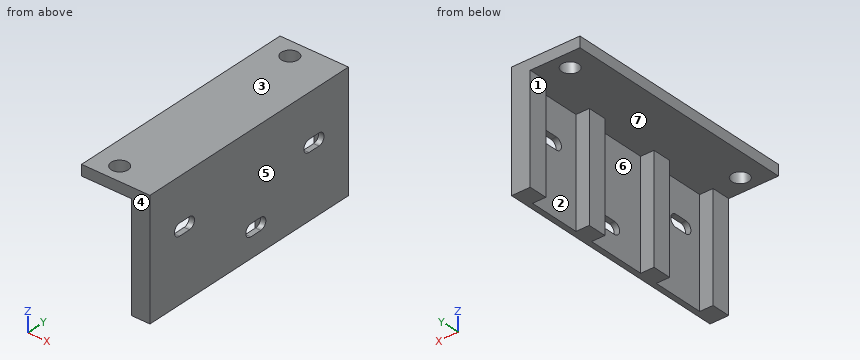
from build123d import *

# Parameters (mm, degrees)
SKETCH1_W           = 25.6624
SKETCH1_H           = 88.9
SKETCH1_R           = 3.175
BOSS_EXTRUDE1_DEPTH = 2
SKETCH2_W           = 2
SKETCH2_H           = 88.9
BOSS_EXTRUDE2_DEPTH = 40
CUT_EXTRUDE1_DEPTH  = 20
SKETCH8_W           = 40
SKETCH8_H           = 7
BOSS_EXTRUDE6_DEPTH = 5
BOSS_EXTRUDE8_START = 2
SKETCH9_W           = 25.6624
SKETCH9_H           = 88.9
SKETCH9_R           = 3.175
BOSS_EXTRUDE8_DEPTH = 2
BOSS_EXTRUDE5_START = 1
SKETCH7_W           = 25.6624
SKETCH7_H           = 88.9
SKETCH7_R           = 3.175
BOSS_EXTRUDE5_DEPTH = 1


with BuildPart() as part:
    # Sketch1 → Boss-Extrude1 (new body)
    with BuildSketch(Plane.XY):
        with Locations((3.8312, 0)):
            Rectangle(SKETCH1_W, SKETCH1_H)
        with Locations((0, -38.1)):
            Circle(SKETCH1_R, mode=Mode.SUBTRACT)
        with Locations((0, 38.1)):
            Circle(SKETCH1_R, mode=Mode.SUBTRACT)
    extrude(amount=-BOSS_EXTRUDE1_DEPTH)

    # Sketch2 → Boss-Extrude2 (add)
    with BuildSketch(Plane(origin=(0, 0, -2), x_dir=(-1, 0, 0), z_dir=(0, 0, -1))):
        with Locations((-15.6624, 0)):
            Rectangle(SKETCH2_W, SKETCH2_H)
    extrude(amount=BOSS_EXTRUDE2_DEPTH)

    # Sketch3 → Cut-Extrude1 (cut)
    with BuildSketch(Plane(origin=(16.6624, 0, 0), x_dir=(0, 0, -1), z_dir=(1, 0, 0))):
        with BuildLine():
            Line((14, -26.75), (14, -31.25))
            ThreePointArc((14, -31.25), (16.25, -33.5), (18.5, -31.25))
            Line((18.5, -31.25), (18.5, -26.75))
            ThreePointArc((18.5, -26.75), (16.25, -24.5), (14, -26.75))
        make_face()
        with BuildLine():
            Line((18.5, 26.75), (18.5, 31.25))
            ThreePointArc((18.5, 31.25), (16.25, 33.5), (14, 31.25))
            Line((14, 31.25), (14, 26.75))
            ThreePointArc((14, 26.75), (16.25, 24.5), (18.5, 26.75))
        make_face()
        with BuildLine():
            Line((30, 5.2), (30, 0.7))
            ThreePointArc((30, 0.7), (32.25, -1.55), (34.5, 0.7))
            Line((34.5, 0.7), (34.5, 5.2))
            ThreePointArc((34.5, 5.2), (32.25, 7.45), (30, 5.2))
        make_face()
    extrude(amount=-CUT_EXTRUDE1_DEPTH, mode=Mode.SUBTRACT)

    # Sketch8 → Boss-Extrude6 (add)
    with BuildSketch(Plane.ZY.offset(-14.6624)):
        with Locations((-22, -14.5)):
            Rectangle(SKETCH8_W, SKETCH8_H)
        with Locations((-22, 14.5)):
            Rectangle(SKETCH8_W, SKETCH8_H)
        with Locations((-22, 40.95)):
            Rectangle(SKETCH8_W, SKETCH8_H)
        with Locations((-22, -40.95)):
            Rectangle(SKETCH8_W, SKETCH8_H)
    extrude(amount=BOSS_EXTRUDE6_DEPTH)

    # Sketch9 → Boss-Extrude8 (add)
    with BuildSketch(Plane.XY.offset(BOSS_EXTRUDE8_START)):
        with Locations((3.8312, 0)):
            Rectangle(SKETCH9_W, SKETCH9_H)
        with Locations((0, -38.1)):
            Circle(SKETCH9_R, mode=Mode.SUBTRACT)
        with Locations((0, 38.1)):
            Circle(SKETCH9_R, mode=Mode.SUBTRACT)
    extrude(amount=-BOSS_EXTRUDE8_DEPTH)

    # Sketch7 → Boss-Extrude5 (add)
    with BuildSketch(Plane.XY.offset(BOSS_EXTRUDE5_START)):
        with Locations((3.8312, 0)):
            Rectangle(SKETCH7_W, SKETCH7_H)
        with Locations((0, -38.1)):
            Circle(SKETCH7_R, mode=Mode.SUBTRACT)
        with Locations((0, 38.1)):
            Circle(SKETCH7_R, mode=Mode.SUBTRACT)
    extrude(amount=-BOSS_EXTRUDE5_DEPTH)


solid = part.part
Could you check a few things on this model? Use its own coordinates, in mm. Face numbers are marked on the shaded views. A direction names the side the tool comes from. Give positions to 0.01 mm unless a question says otherwise; leave off trailing zeros. Order: outer loops, then holes, each group sorted by start corner. A loop starts at its lowest first (then second) coordinate and runs counter-clockwise, first axis right, second up. Notation, with made-up numbers: (66.25, 61) - (103.25, 61) arc R25 ccw to (103.25, 94) - close; hole circle Ø9 at (29, 63.5). An arc over 180 degrees is marked (long way). One line per item, written item: value. Start each with the question number.
1. For P1, Ø2, axis at y = -16, z = -12.5, coming from the -X side; P2, Ø1.5, axis at y = 23.5, z = -20, coming from the -X side; P3, Ø10, axis at x = 0, y = 38.1, coming from the -Z side, each with a flat end and sliding along its axis, tell me the tip position at first contact or that it passes through.
2. Imagine slicing it at C-C on z = -29. List the corners of the cut face in (x, y) for me.
3. Imagine slicing it at A-A on z = -16.25. List the corners of the cut face in (x, y) for me.
4. Thinking about a two-plate mould opening in Y: for the marked faces 4, 5, 6 and 7, which applies, +Y half, -Y half, draft (parallel to the pull), parting line (faces both ways), or undercut?
5. Imagine slicing it at D-D on x = 5. List the corners of the cut face in (y, z) for me, plus the area to 3 significant figures.
6. Imagine slicing it at B-B on y = -16.5. List the corners of the cut face in (x, z) for me, plus the area to 3 significant figures.
7. If I drill on probe 1 along Y at (x, z) = (0, -0.4) (3 decimals); probe 2 along Y at (x, z) = (12, -19.5); probe 3 along Y at (x, z) = (-0.5, -1), over which ranges is the centre line in solid material (lowest first)?
8. For the marked faces 1, 2 and 3, which set-ups out of +Z, -Z, +X, -X, +Y, -Y let a thin tool reach every point of the face, with its end or its side?
Values:
1. P1: x = 9.66
1. P2: x = 14.66
1. P3: z = -2
2. outline: (9.66, -44.45) - (16.66, -44.45) - (16.66, 44.45) - (9.66, 44.45) - (9.66, 37.45) - (14.66, 37.45) - (14.66, 18) - (9.66, 18) - (9.66, 11) - (14.66, 11) - (14.66, -11) - (9.66, -11) - (9.66, -18) - (14.66, -18) - (14.66, -37.45) - (9.66, -37.45) - close
3. outline: (9.66, -44.45) - (16.66, -44.45) - (16.66, -33.5) - (14.66, -33.5) - (14.66, -37.45) - (9.66, -37.45) - close; (9.66, -18) - (14.66, -18) - (14.66, -24.5) - (16.66, -24.5) - (16.66, 24.5) - (14.66, 24.5) - (14.66, 18) - (9.66, 18) - (9.66, 11) - (14.66, 11) - (14.66, -11) - (9.66, -11) - close; (9.66, 37.45) - (14.66, 37.45) - (14.66, 33.5) - (16.66, 33.5) - (16.66, 44.45) - (9.66, 44.45) - close
4. face 4: -Y half
4. face 5: draft
4. face 6: undercut
4. face 7: undercut
5. outline: (-44.45, -2) - (44.45, -2) - (44.45, 2) - (-44.45, 2) - close
5. area: 356 mm²
6. outline: (-9, -2) - (9.66, -2) - (9.66, -42) - (16.66, -42) - (16.66, 2) - (-9, 2) - close
6. area: 383 mm²
7. probe 1: -44.45 to -41.275, -34.925 to 34.925, 41.275 to 44.45
7. probe 2: -44.45 to -37.45, -18 to -11, 11 to 18, 37.45 to 44.45
7. probe 3: -44.45 to -41.24, -34.96 to 34.96, 41.24 to 44.45
8. face 1: -Z, -X, +Y, -Y
8. face 2: -Z, -X
8. face 3: +Z, +X, -X, +Y, -Y
